Part model, mm, in its own coordinate system. Face numbers are marked on the shaded views. Round coordinates to 2 decimals unless told otherwise and drop trailing zeros. Write each loop counter-clockwise with the first axis right and the second up, starting at its lowest first coordinate (ties: lowest second). Pieces come first, ordered by that corner, then holes.
```python
from build123d import *

# Parameters (mm, degrees)
SKETCH1_W           = 11.5
SKETCH1_H           = 13.5
SKETCH1_W_2         = 1
SKETCH1_H_2         = 11
SKETCH1_W_3         = 3
SKETCH1_H_3         = 1
BOSS_EXTRUDE1_DEPTH = 1
CUT_EXTRUDE1_DEPTH  = 11.325938214
SKETCH3_W           = 2.5
SKETCH3_H           = 10.5
BOSS_EXTRUDE2_DEPTH = 3


with BuildPart() as part:
    # Sketch1 → Boss-Extrude1 (new body)
    with BuildSketch(Plane.XY):
        Rectangle(SKETCH1_W, SKETCH1_H)
        with Locations((6.25, -1.25)):
            Rectangle(SKETCH1_W_2, SKETCH1_H_2)
        with Locations((4.25, 7.25)):
            Rectangle(SKETCH1_W_3, SKETCH1_H_3)
    extrude(amount=-BOSS_EXTRUDE1_DEPTH)

    # Sketch2 → Cut-Extrude1 (cut, through all)
    with BuildSketch(Plane.XY):
        Polygon((6.75, 4.25), (5.75, 4.25), (5.75, 7.75), (2.75, 7.75), (2.75, 6.75), (-5.75, 6.75), (-5.75, -6.75), (6.75, -6.75), (6.75, -6.5), (6.5, -6.5), (-5.5, -6.5), (-5.5, 6.5), (3, 6.5), (3, 7.5), (5.5, 7.5), (5.5, 4), (6.5, 4), (6.75, 4), align=None)
    extrude(amount=-CUT_EXTRUDE1_DEPTH, mode=Mode.SUBTRACT)

    # Sketch3 → Boss-Extrude2 (add)
    with BuildSketch(Plane(origin=(0, 0, 0), x_dir=(-1, 0, 0), z_dir=(0, 0, -1))):
        with Locations((-5.5, -1.25)):
            Rectangle(SKETCH3_W, SKETCH3_H)
    extrude(amount=BOSS_EXTRUDE2_DEPTH)


solid = part.part
```
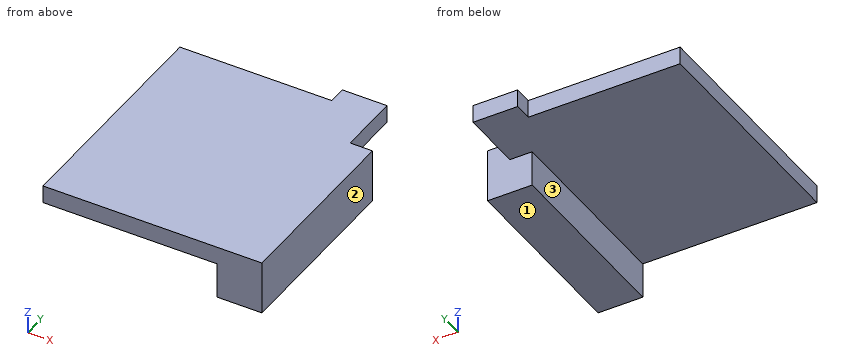
Q1. Cut at A-A on x = 4.75. Write the cut outline in (y, z), plus the area to 3 significant figures.
Values follow:
outline: (-6.5, -3) - (4, -3) - (4, -1) - (7.5, -1) - (7.5, 0) - (-6.5, 0) - close
area: 35.0 mm2
Q2. Cut at B-B on y = -4.75. Write the cut outline in (x, z).
Values follow:
outline: (-5.5, -1) - (4.25, -1) - (4.25, -3) - (6.75, -3) - (6.75, 0) - (-5.5, 0) - close
Q3. Mould opens along X. For the marked faces 1, 2 and 3 say: +X half, -X half, draft (parallel to the pull), parting line (faces both ways), or undercut.
Values follow:
face 1: draft
face 2: +X half
face 3: -X half
Q4. Cut at D-D on y = 6. Write the cut outline in (x, z), plus the area to 3 significant figures.
Values follow:
outline: (-5.5, -1) - (5.5, -1) - (5.5, 0) - (-5.5, 0) - close
area: 11.0 mm2
Q5. Wall check: L1, parallel to X at y = -2.25, z = -1.7; L2, parallel to Z at x = -1.5, y = 2.75; L3, parallel to Y at x = 5.75, z = -2.35. Give the ranges that are in metal, low to high.
Values follow:
L1: x = 4.25 to 6.75
L2: z = -1 to 0
L3: y = -6.5 to 4
Q6. Cut at C-C on z = -1.6. Write the cut outline in (x, y).
Values follow:
outline: (4.25, -6.5) - (6.75, -6.5) - (6.75, 4) - (4.25, 4) - close
Q7. Drop flat-ended pins along their axis: pin 1 (0.8 mm diameter, centred on y = 5, z = -0.5, fed in from +X); pin 2 (1 mm diameter, centred on x = -3, y = 0.5, fed in from -Z). Give the stop position or say it passes through.
Values follow:
pin 1: stops at x = 5.5
pin 2: stops at z = -1
